The listing builds one solid part. Answer for the finished solid, in the listing's coordinates (mm). A direction names the side the tool comes from. Coordinates: 2 decimals unless noted, no trailing zeros. Order: outer loops, then holes, each group sorted by start corner. A loop starts at its lowest first (then second) coordinate and runs counter-clockwise, first axis right, second up. Notation, with made-up numbers: (81, 39.25) -> (123, 39.25) arc R14 cw to (123, 47.25) -> close; hole circle Ø1 at (-8.5, 82). An arc over 180 degrees is marked (long way). Answer in a Markdown table with one row per item.
Autodesk Inventor part; units mm, degrees
ref_plane "Work Plane1" through (0, 0, 0) normal (0, 0, 1) x (1, 0, 0)
ref_plane "YZ Plane" through (0, 0, 0) normal (1, 0, 0) x (0, 1, 0)
ref_plane "XZ Plane" through (0, 0, 0) normal (0, 1, 0) x (-1, 0, 0)
ref_plane "Work Plane1" through (0, 0, 0) normal (0, 0, 1) x (1, 0, 0)
sketch "Sketch1" plane through (0, 0, 0) normal (0, 0, 1) x (1, 0, 0)
  arc A0 (-113.2188, 0) -> (-109.7581, 3.4607) centre (-113.2188, 3.4607) ccw
  line L0 (-109.7581, 17.1767) -> (-109.7581, 3.4607)
  arc A1 (-109.7581, 17.1767) -> (-114.8063, 22.225) centre (-114.8063, 17.1767) ccw
  line L1 (-115.8223, 22.225) -> (-114.8063, 22.225)
  arc A2 (-115.8223, 22.225) -> (-119.2831, 18.7642) centre (-115.8223, 18.7642) ccw
  line L2 (-119.2831, 16.4211) -> (-119.2831, 18.7642)
  arc A3 (-119.2831, 16.4211) -> (-116.6161, 16.4211) centre (-117.9496, 16.4211) ccw
  line L3 (-116.6161, 18.7642) -> (-116.6161, 16.4211)
  arc A4 (-115.8223, 19.558) -> (-116.6161, 18.7642) centre (-115.8223, 18.7642) ccw
  line L4 (-114.8063, 19.558) -> (-115.8223, 19.558)
  arc A5 (-112.4251, 17.1767) -> (-114.8063, 19.558) centre (-114.8063, 17.1767) ccw
  line L5 (-112.4251, 3.4607) -> (-112.4251, 17.1767)
  arc A6 (-113.2188, 2.667) -> (-112.4251, 3.4607) centre (-113.2188, 3.4607) ccw
  line L6 (-147.5723, 2.667) -> (-113.2188, 2.667)
  arc A7 (-148.3661, 3.4607) -> (-147.5723, 2.667) centre (-147.5723, 3.4607) ccw
  line L7 (-148.3661, 17.1767) -> (-148.3661, 3.4607)
  arc A8 (-145.9848, 19.558) -> (-148.3661, 17.1767) centre (-145.9848, 17.1767) ccw
  line L8 (-144.9688, 19.558) -> (-145.9848, 19.558)
  arc A9 (-144.1751, 18.7642) -> (-144.9688, 19.558) centre (-144.9688, 18.7642) ccw
  line L9 (-144.1751, 16.4211) -> (-144.1751, 18.7642)
  arc A10 (-144.1751, 16.4211) -> (-141.5081, 16.4211) centre (-142.8416, 16.4211) ccw
  line L10 (-141.5081, 18.7642) -> (-141.5081, 16.4211)
  arc A11 (-141.5081, 18.7642) -> (-144.9688, 22.225) centre (-144.9688, 18.7642) ccw
  line L11 (-145.9848, 22.225) -> (-144.9688, 22.225)
  arc A12 (-145.9848, 22.225) -> (-151.0331, 17.1767) centre (-145.9848, 17.1767) ccw
  line L12 (-151.0331, 3.4607) -> (-151.0331, 17.1767)
  arc A13 (-151.0331, 3.4607) -> (-147.5723, 0) centre (-147.5723, 3.4607) ccw
  line L13 (-113.2188, 0) -> (-147.5723, 0)
  point P0 (0, 0)
extrude "Extrusion1" add sketch "Sketch1" along normal blind 381
properties part number "Unistrut 15"
(1) Which of the six approach directions +Z, -Z, +X, -X, +Y, -Y give full straight-line access (tool end or side, diameter ignored) to faces 5 (the flat face through (-148.366, 10, 188)), 6 (the flat face through (-130, 2, 381))?
Check values:
| item | result |
|---|---|
| face 5 | +Z, -Z |
| face 6 | +Z, +X, -X, +Y, -Y |
(2) A flat-ended cylindrical pin translates along its axis: pin 1 (1.9 mm diameter, centred on y = 17.5, z = 264, fed in from +X). Find the tip coordinate at first contact, or state that the pin passes through.
Check values:
| item | result |
|---|---|
| pin 1 | x = -109.76 |
(3) Find the intervals of material crossed by line 1 along X through (y, z) = (16.5, 251); line 2 along X through (y, z) = (16, 154); line 3 along X through (y, z) = (14.25, 137.5), in increasing order. Write a range as from..to.
Check values:
| item | result |
|---|---|
| line 1 | -151.03..-148.37, -144.18..-141.51, -119.28..-116.62, -112.43..-109.76 |
| line 2 | -151.03..-148.37, -144.11..-141.58, -119.21..-116.68, -112.43..-109.76 |
| line 3 | -151.03..-148.37, -112.43..-109.76 |
(4) A cutting plane is placed at B-B, the plane z = 231. Determine the outline of the cut face in (x, y) (1 decimal), then the cut area to 3 significant figures.
Check values:
| item | result |
|---|---|
| outline | (-151, 3.5) arc R3.5 ccw to (-147.6, 0) -> (-113.2, 0) arc R3.5 ccw to (-109.8, 3.5) -> (-109.8, 17.2) arc R5 ccw to (-114.8, 22.2) -> (-115.8, 22.2) arc R3.5 ccw to (-119.3, 18.8) -> (-119.3, 16.4) arc R1.3 ccw to (-116.6, 16.4) -> (-116.6, 18.8) arc R0.8 cw to (-115.8, 19.6) -> (-114.8, 19.6) arc R2.4 cw to (-112.4, 17.2) -> (-112.4, 3.5) arc R0.8 cw to (-113.2, 2.7) -> (-147.6, 2.7) arc R0.8 cw to (-148.4, 3.5) -> (-148.4, 17.2) arc R2.4 cw to (-146, 19.6) -> (-145, 19.6) arc R0.8 cw to (-144.2, 18.8) -> (-144.2, 16.4) arc R1.3 ccw to (-141.5, 16.4) -> (-141.5, 18.8) arc R3.5 ccw to (-145, 22.2) -> (-146, 22.2) arc R5 ccw to (-151, 17.2) -> close |
| area | 255 mm² |
(5) For a pull along X with two mould halves and no side action, classify faces 1 (the flat face through (-109.758, 10, 188)), 2 (the flat face through (-130, 0, 188)), 3 (the flat face through (-112.425, 10, 188)), 4 (the flat face through (-131, 2.667, 188)) as released by +X, released by -X, zero draft, split by the parting line, or undercut.
Check values:
| item | result |
|---|---|
| face 1 | released by +X |
| face 2 | zero draft |
| face 3 | undercut |
| face 4 | undercut |
(6) A cutting plane is placed at A-A, the plane y = 7.25. Determine the outline of the cut face in (x, z).
Check values:
| item | result |
|---|---|
| outline | (-151.03, 0) -> (-148.37, 0) -> (-148.37, 381) -> (-151.03, 381) -> close; (-112.43, 0) -> (-109.76, 0) -> (-109.76, 381) -> (-112.43, 381) -> close |
